Design review of the part shown in the three views and the two pictorial views. Dimensions are in mm from the part's minimum x, y and z. A direction names the side the tool comes from. Round coordinates to 2 decimals unless told otherwise and drop trailing zeros. Loops run counter-clockwise (first coordinate to the right, second up) from the corner with the lowest first, then second, coordinate; pieces in that order, holes last. Notation, with made-up numbers: (6, 59) - (21, 59) arc R15 cw to (21, 80) - close; hole circle Ø9 at (11, -10.75). An arc over 180 degrees is marked (long way). Return JSON: item names as keys, results as strings. Group by question number.
(1) We need section B-B, the plane x = 85.5. Write out the cut boundary in (y, z).
(2) We need section C-C, the plane y = 72. Write out the cut boundary in (x, z), and give its area (3 significant figures).
(3) We need section A-A, the plane y = 16. Write out the cut boundary in (x, z).
(4) We need section D-D, the plane z = 34. Write out the cut boundary in (x, y), and give its area (3 significant figures).
(5) The part is to be moulded in two halves that separate along Z. For the marked faces 3, 4 and 5, say which applies: pulls with the +Z half, pulls with the -Z half, needs draft (parallel to the pull), parting line crosses it, or undercut.
(6) Clearance check with flat-ended pins moving along their axes: pin 1 (1 mm diameter, centred on y = 59.5, z = 31, fed in from -X); pin 2 (4 mm diameter, centred on x = 57.5, z = 41.5, fed in from -Y) (1 decimal); pin 3 (3 mm diameter, centred on x = 41.5, z = 41.5, fed in from +Y) (1 decimal). State where each tip first meets the part, or that it passes through.
(7) For the marked faces 1 and 2, list the 3-axis set-ups (+Z, -Z, +X, -X, +Y, -Y) from which the entire face can be reached by the end or side of a thin tool; tool diameter is ignored.
(8) Wall thickness on L1, parallel to Z at x = 153, y = 61 (1 decimal); L2, parallel to Z at x = 177.5, y = 74.5 (1 decimal); L3, parallel to Y at x = 186, z = 32 (1 decimal): over which ranges is each line inside the solid? List them lowest first. Write a range as [from, to].
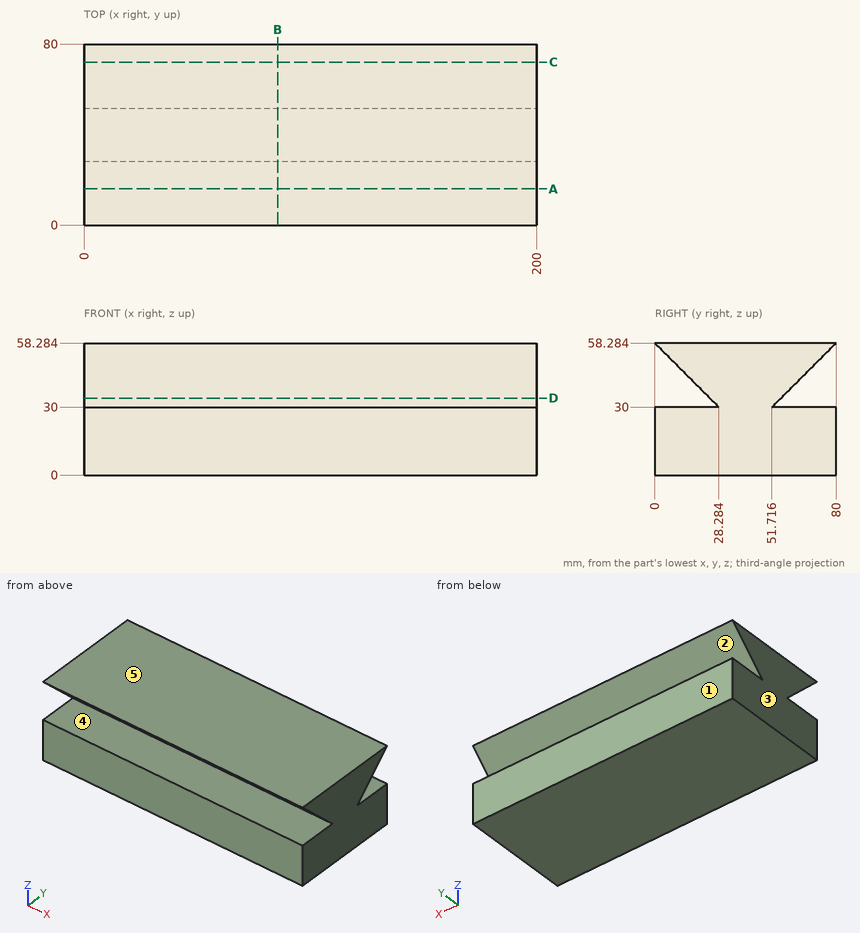
Solutions:
{
 "1": {"outline": "(0, 0) - (80, 0) - (80, 30) - (51.72, 30) - (80, 58.28) - (0, 58.28) - (28.28, 30) - (0, 30) - close"},
 "2": {"outline": "(0, 0) - (200, 0) - (200, 30) - (0, 30) - close; (0, 50.28) - (200, 50.28) - (200, 58.28) - (0, 58.28) - close", "area": "7,600 mm^2"},
 "3": {"outline": "(0, 0) - (200, 0) - (200, 30) - (0, 30) - close; (0, 42.28) - (200, 42.28) - (200, 58.28) - (0, 58.28) - close"},
 "4": {"outline": "(0, 24.28) - (200, 24.28) - (200, 55.72) - (0, 55.72) - close", "area": "6,290 mm^2"},
 "5": {"face 3": "needs draft", "face 4": "undercut", "face 5": "pulls with the +Z half"},
 "6": {"pin 1": "through", "pin 2": "y = 14.8", "pin 3": "y = 64.7"},
 "7": {"face 1": "+Z, -Z, +X, -X, +Y", "face 2": "+X, -X, +Y"},
 "8": {"L1": "[0, 30], [39.3, 58.3]", "L2": "[0, 30], [52.8, 58.3]", "L3": "[26.3, 53.7]"}
}
